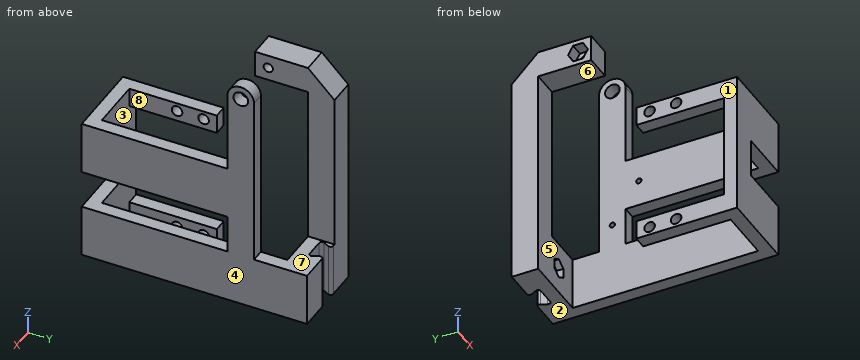
from build123d import *

# Parameters (mm, degrees)
ESBO_O1_W                   = 5
ESBO_O1_H                   = 33
RESSALTO_EXTRUS_O1_DEPTH    = 80
ESBO_O2_W                   = 40
ESBO_O2_H                   = 33
ESBO_O2_W_2                 = 25.6
CORTE_EXTRUS_O1_DEPTH       = 19
ESBO_O4_R                   = 2
CORTE_EXTRUS_O3_DEPTH       = 12
ESBO_O5_W                   = 10
ESBO_O5_H                   = 20
RESSALTO_EXTRUS_O2_DEPTH    = 10
ESBO_O6_R                   = 1.75
CORTE_EXTRUS_O4_DEPTH       = 15
CORTE_EXTRUS_O5_DEPTH       = 5
ESBO_O8_R                   = 5
ESBO_O8_R_2                 = 2.75
RESSALTO_EXTRUS_O3_DEPTH    = 5
ESBO_O9_W                   = 20
ESBO_O9_H                   = 20
ESBO_O9_W_2                 = 25
ESBO_O9_H_2                 = 10
CORTE_EXTRUS_O6_DEPTH       = 25.6
CORTE_EXTRUS_O7_START       = -20
ESBO_O11_W                  = 34.4
ESBO_O11_H                  = 20
ESBO_O11_W_2                = 14.4
ESBO_O11_H_2                = 60
CORTE_EXTRUS_O7_DEPTH       = 20
ESBO_O12_R                  = 1.75
CORTE_EXTRUS_O8_DEPTH       = 25
CORTE_EXTRUS_O9_DEPTH       = 2.5
FILETE1_R                   = 1
FILETE2_R                   = 1
CORTE_EXTRUS_O10_DEPTH      = 74
CORTE_EXTRUS_O10_DEPTH_BACK = 84
ESBO_O14_W                  = 30
ESBO_O14_H                  = 90
ESBO_O15_W                  = 30
ESBO_O15_H                  = 5
CORTE_EXTRUS_O11_DEPTH      = 120
ESBO_O16_R                  = 1
CORTE_EXTRUS_O12_DEPTH      = 2


with BuildPart() as part:
    # Esboço1 → Ressalto-extrusão1 (new body)
    with BuildSketch(Plane.XY):
        Polygon((-2.5, 45), (-15, 45), (-15, 35), (-10, 35), (15, 35), (15, 45), (2.5, 45), (5, 40), (-5, 40), align=None)
        Polygon((-10, 35), (-15, 35), (-15, -45), (-10, -45), (-10, -35), align=None)
        Polygon((-10, -35), (-10, -45), (15, -45), (15, -35), (10, -35), align=None)
        with Locations((12.5, -18.5)):
            Rectangle(ESBO_O1_W, ESBO_O1_H)
    extrude(amount=RESSALTO_EXTRUS_O1_DEPTH)

    # Esboço2 → Corte-extrusão1 (cut)
    with BuildSketch(Plane(origin=(15, 0, 0), x_dir=(0, 0, -1), z_dir=(1, 0, 0))):
        with Locations((-27.2, -18.5)):
            Rectangle(ESBO_O2_W, ESBO_O2_H)
        with Locations((-67.2, -18.5)):
            Rectangle(ESBO_O2_W_2, ESBO_O2_H)
    extrude(amount=-CORTE_EXTRUS_O1_DEPTH, mode=Mode.SUBTRACT)

    # Esboço4 → Corte-extrusão3 (cut)
    with BuildSketch(Plane.ZY.offset(-10)):
        with Locations(Location((3.104223841, -7.000828192, 0), (0, 0, 270))):
            Circle(ESBO_O4_R)
        with Locations(Location((3.104223841, -17.002484575, 0), (0, 0, 270))):
            Circle(ESBO_O4_R)
        with Locations(Location((51.210481376, -17.002484575, 0), (0, 0, 270))):
            Circle(ESBO_O4_R)
        with Locations(Location((51.210481376, -7.000828192, 0), (0, 0, 270))):
            Circle(ESBO_O4_R)
    extrude(amount=-CORTE_EXTRUS_O3_DEPTH, mode=Mode.SUBTRACT)

    # Esboço5 → Ressalto-extrusão2 (add)
    with BuildSketch(Plane(origin=(15, 0, 0), x_dir=(0, 0, -1), z_dir=(1, 0, 0))):
        with Locations((-85, 25)):
            Rectangle(ESBO_O5_W, ESBO_O5_H)
        Polygon((-90, 35), (-80, 45), (-80, 35), align=None)
    extrude(amount=-RESSALTO_EXTRUS_O2_DEPTH)

    # Esboço6 → Corte-extrusão4 (cut)
    with BuildSketch(Plane(origin=(15, 0, 0), x_dir=(0, 0, -1), z_dir=(1, 0, 0))):
        with Locations(Location((-85, 20, 0), (0, 0, 90))):
            Circle(ESBO_O6_R)
    extrude(amount=-CORTE_EXTRUS_O4_DEPTH, mode=Mode.SUBTRACT)

    # Esboço7 → Corte-extrusão5 (cut)
    with BuildSketch(Plane(origin=(15, 0, 0), x_dir=(0, 0, -1), z_dir=(1, 0, 0))):
        Polygon((-81.75, 21.876388375), (-85, 23.75277675), (-88.25, 21.876388375), (-88.25, 18.123611625), (-85, 16.24722325), (-81.75, 18.123611625), align=None)
    extrude(amount=-CORTE_EXTRUS_O5_DEPTH, mode=Mode.SUBTRACT)

    # Esboço8 → Ressalto-extrusão3 (add)
    # profile 1 of 3: a face of its own
    with BuildSketch(Plane.ZY.offset(15)):
        with BuildLine():
            Line((80, 25), (80, 20.00000004))
            ThreePointArc((80, 20.00000004), (81.464466108, 23.53553392), (85, 25))
            Line((85, 25), (80, 25))
        make_face()
    # profile 2 of 3: a face of its own
    with BuildSketch(Plane.ZY.offset(15)):
        with Locations((85, 20)):
            Circle(ESBO_O8_R)
        with Locations(Location((85, 20, 0), (0, 0, 270))):
            Circle(ESBO_O8_R_2, mode=Mode.SUBTRACT)
    # profile 3 of 3: a face of its own
    with BuildSketch(Plane.ZY.offset(15)):
        with BuildLine():
            Line((80, 15), (85, 15))
            ThreePointArc((85, 15), (81.46446608, 16.464466108), (80, 20.00000004))
            Line((80, 20.00000004), (80, 15))
        make_face()
    extrude(amount=-RESSALTO_EXTRUS_O3_DEPTH)

    # Esboço9 → Corte-extrusão6 (cut)
    with BuildSketch(Plane.XY.offset(80)):
        with Locations((-5, 35)):
            Rectangle(ESBO_O9_W, ESBO_O9_H)
        Polygon((-15, 15), (-15, -45), (-10, -45), (-10, -35), (-10, 15), align=None)
        with Locations((2.5, -40)):
            Rectangle(ESBO_O9_W_2, ESBO_O9_H_2)
    extrude(amount=-CORTE_EXTRUS_O6_DEPTH, mode=Mode.SUBTRACT)

    # Esboço11 → Corte-extrusão7 (cut)
    with BuildSketch(Plane.ZY.offset(15).offset(CORTE_EXTRUS_O7_START)):
        with Locations((37.2, 35)):
            Rectangle(ESBO_O11_W, ESBO_O11_H)
        with Locations((27.2, -15)):
            Rectangle(ESBO_O11_W_2, ESBO_O11_H_2)
    extrude(amount=CORTE_EXTRUS_O7_DEPTH, mode=Mode.SUBTRACT)

    # Esboço12 → Corte-extrusão8 (cut)
    with BuildSketch(Plane(origin=(0, 40, 0), x_dir=(1, 0, 0), z_dir=(0, 1, 0))):
        with Locations(Location((0, -10, 0), (0, 0, 270))):
            Circle(ESBO_O12_R)
    extrude(amount=-CORTE_EXTRUS_O8_DEPTH, mode=Mode.SUBTRACT)

    # Esboço13 → Corte-extrusão9 (cut)
    with BuildSketch(Plane.XZ.offset(-35)):
        Polygon((0, 6.24722325), (3.25, 8.123611625), (3.25, 11.876388375), (0, 13.75277675), (-3.25, 11.876388375), (-3.25, 8.123611625), align=None)
    extrude(amount=-CORTE_EXTRUS_O9_DEPTH, mode=Mode.SUBTRACT)

    # Filete1
    filete1_edges = [part.edges().sort_by_distance(p)[0] for p in [
        (2.5, 45, 10),
        (-2.5, 45, 10),
    ]]
    fillet(filete1_edges, radius=FILETE1_R)

    # Filete2
    filete2_edges = [part.edges().sort_by_distance(p)[0] for p in [
        (-5, 40, 10),
        (5, 40, 10),
    ]]
    fillet(filete2_edges, radius=FILETE2_R)

    # Espelhar1: part across plane


with BuildPart() as part_1:
    add(part.part)
    add(part.part.mirror(Plane(origin=(15, 0, 80), x_dir=(0, 0, 1), z_dir=(1, 0, 0))))

    # Esboço14 → Corte-extrusão10 (cut, two sides: drawn at the far end of the back side and taken through both)
    with BuildSketch(Plane.XY.offset(54.4).offset(-CORTE_EXTRUS_O10_DEPTH_BACK)):
        Rectangle(ESBO_O14_W, ESBO_O14_H)
    extrude(amount=CORTE_EXTRUS_O10_DEPTH + CORTE_EXTRUS_O10_DEPTH_BACK, mode=Mode.SUBTRACT)

    # Esboço15 → Corte-extrusão11 (cut)
    with BuildSketch(Plane.XY.offset(54.4)):
        with Locations((30, -42.5)):
            Rectangle(ESBO_O15_W, ESBO_O15_H)
    extrude(amount=-CORTE_EXTRUS_O11_DEPTH, mode=Mode.SUBTRACT)

    # Esboço16 → Corte-extrusão12 (cut)
    with BuildSketch(Plane.ZY.offset(-40)):
        with Locations(Location((29.4, 20, 0), (0, 0, 270))):
            Circle(ESBO_O16_R)
        with Locations(Location((44.4, 10, 0), (0, 0, 270))):
            Circle(ESBO_O16_R)
    extrude(amount=-CORTE_EXTRUS_O12_DEPTH, mode=Mode.SUBTRACT)


solid = part_1.part
Design review of the part built by this model. Coordinates are the model's own, in mm. Face numbers are marked on the shaded views. A direction names the side the tool comes from. Round coordinates to 2 decimals unless told otherwise and drop trailing zeros. Write each loop counter-clockwise with the first axis right and the second up, starting at its lowest first coordinate (ties: lowest second). Pieces come first, ordered by that corner, then holes.
Item 1: Consider section B-B on y = 7.5. Give the boundary of the cut face in (x, z), and give its area (3 significant figures).
Item 2: For pin 1 Ø3 at (y, z) = (-7, 51.21) entering from -X; pin 2 Ø3 at (x, y) = (18, 19.5) entering from -Z; pin 3 Ø5.5 at (x, z) = (41.5, 25.5) entering from -Y; pin 4 Ø1.5 at (x, y) = (37.5, -5.5) entering from -Z, all flat-tipped, find the tip position at first contact; note any pin that passes through.
Item 3: Wall thickness on L1, parallel to Y at x = 27.5, z = 15; L2, parallel to Z at x = 30, y = 38; L3, parallel to X at y = -30.5, z = 48.5: over which ranges is each line inside the solid? List them lowest first.
Item 4: Consider section D-D on z = 33. Give the boundary of the cut face in (x, y).
Item 5: For the marked faces 4, 5, 6, 7 and 8, list the 3-axis set-ups (+Z, -Z, +X, -X, +Y, -Y) from which the entire face can be reached by the end or side of a thin tool; tool diameter is ignored.
Item 6: Consider section C-C on z = 10. Give the boundary of the cut face in (x, y), and give its area (4 significant figures).
Item 7: Draft analysis for pull direction X (two halves, no side actions). For the marked faces 1, 2 and 3, state which applies: released by +X, released by -X, zero draft, split by the parting line, or undercut.
Item 8: Consider section A-A on x = 23.5. Give the boundary of the cut face in (y, z), and give its area (3 significant figures).
Check values:
1. outline: (40, 0) - (45, 0) - (45, 20) - (40, 20) - close; (40, 34.4) - (45, 34.4) - (45, 54.4) - (40, 54.4) - close
1. area: 200 mm2
2. pin 1: stops at x = 40
2. pin 2: stops at z = 80
2. pin 3: stops at y = 15
2. pin 4: passes through
3. L1: y = -40 to -35, 35 to 40
3. L2: z = 0 to 8.25, 11.75 to 20
3. L3: x = 15 to 20, 40 to 45
4. outline: (15, -40) - (25, -40) - (25, -35) - (15, -35) - close; (15, 35) - (25, 35) - (25, 45) - (15, 45) - close; (40, 15) - (45, 15) - (45, 25) - (40, 25) - close
5. face 4: +Z, -Z, +X, +Y, -Y
5. face 5: -Z, -X
5. face 6: -Z, -X, -Y
5. face 7: +Z, +X, +Y
5. face 8: +Z, -Z
6. outline: (15, -40) - (45, -40) - (45, 45) - (34.12, 45) arc R1 ccw to (33.22, 43.55) - (34.28, 41.45) arc R1 cw to (33.38, 40) - (31.75, 40) - (31.75, 37.5) - (33.25, 37.5) - (33.25, 35) - (40, 35) - (40, -35) - (15, -35) - close; (15, 35) - (26.75, 35) - (26.75, 37.5) - (28.25, 37.5) - (28.25, 40) - (26.62, 40) arc R1 cw to (25.72, 41.45) - (26.78, 43.55) arc R1 ccw to (25.88, 45) - (15, 45) - close
6. area: 737.5 mm2
7. face 1: released by -X
7. face 2: zero draft
7. face 3: undercut
8. outline: (-40, 0) - (-35, 0) - (-35, 54.4) - (-40, 54.4) - close; (15, 80) - (35, 80) - (35, 0) - (45, 0) - (45, 80) - (35, 90) - (15, 90) - close; hole circle Ø3.5 at (20, 85)
8. area: 1,310 mm2
